Verification items for this drawing (mm, ordinates from the low corner). Round coordinates to 2 decimals unless told otherwise and drop trailing zeros. Write each loop counter-clockwise with the first axis right and the second up, starting at its lowest first coordinate (ties: lowest second). Pieces come first, ordered by that corner, then holes. Notation, with made-up numbers: (70, 71.5) -> (107, 71.5) arc R10 ccw to (107, 78.5) -> close; hole circle Ø10 at (72.5, -8). An arc over 180 degrees is marked (long way). Return JSON: item names as keys, results as strings. Group by question number.
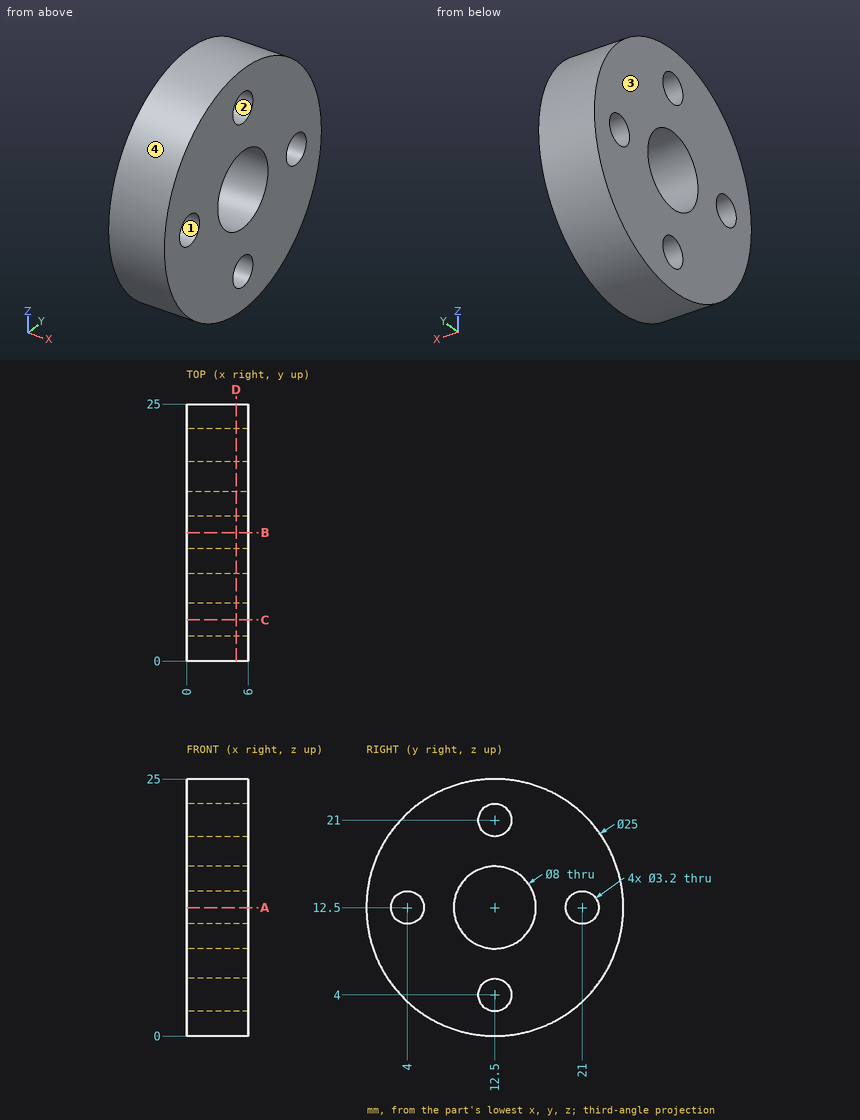
1) Sectioned sample at A-A on z = 12.5. Enter the section's corners in (x, y).
2) Sectioned sample at C-C on y = 4. Enter the section's corners in (x, z).
3) Mould release check, pull along Z, two halves, no side actions. Record for the marked faces 1, 2, 3 and 4: +Z half, -Z half, draft (parallel to the pull), parting line (faces both ways), or undercut.
4) Sectioned sample at D-D on x = 4.8. Enter the section's corners in (y, z), and give its area (3 significant figures).
5) Go/stop test with flat-tipped pins: P1, Ø3, axis at x = 3, z = 4, coming from the -Y side; P2, Ø7, axis at y = 12.5, z = 12.5, coming from the -X side. Record where each tip stops, or that it passes through.
6) Material ranges on probe 1 along Z at (x, y) = (2.15, 12.5); probe 2 along Y at (x, z) = (4.75, 13); probe 3 along Z at (x, y) = (3.15, 21), recorded low to high. Write a range as [from, to].
Evaluation:
{
 "1": {"outline": "(0, 0) -> (6, 0) -> (6, 2.4) -> (0, 2.4) -> close; (0, 5.6) -> (6, 5.6) -> (6, 8.5) -> (0, 8.5) -> close; (0, 16.5) -> (6, 16.5) -> (6, 19.4) -> (0, 19.4) -> close; (0, 22.6) -> (6, 22.6) -> (6, 25) -> (0, 25) -> close"},
 "2": {"outline": "(0, 3.33) -> (6, 3.33) -> (6, 10.9) -> (0, 10.9) -> close; (0, 14.1) -> (6, 14.1) -> (6, 21.67) -> (0, 21.67) -> close"},
 "3": {"face 1": "undercut", "face 2": "undercut", "face 3": "draft", "face 4": "parting line"},
 "4": {"outline": "circle Ø25 at (12.5, 12.5); hole circle Ø3.2 at (4, 12.5); hole circle Ø8 at (12.5, 12.5); hole circle Ø3.2 at (12.5, 4); hole circle Ø3.2 at (12.5, 21); hole circle Ø3.2 at (21, 12.5)", "area": "408 mm2"},
 "5": {"P1": "stops at y = 2.14", "P2": "passes through"},
 "6": {"probe 1": "z = [0, 2.4], [5.6, 8.5], [16.5, 19.4], [22.6, 25]", "probe 2": "y = [0.01, 2.48], [5.52, 8.53], [16.47, 19.48], [22.52, 24.99]", "probe 3": "z = [3.33, 10.9], [14.1, 21.67]"}
}
